Here's how the part is built. I have some questions about the finished solid (model axes, mm). Face numbers are marked on the shaded views. A direction names the side the tool comes from. Coordinates: 2 decimals unless noted, no trailing zeros. Answer in a Markdown table with one row per item. Add a question column.
Item 1: I'm going to push flat-ended pins straight in: pin 1 (1.5 mm diameter, centred on x = -9.5, z = -2.5, fed in from -Y); pin 2 (1 mm diameter, centred on y = 6.5, z = 1.5, fed in from +X); pin 3 (18 mm diameter, centred on x = 0, y = 0, fed in from -Z); pin 4 (2 mm diameter, centred on y = 20.5, z = 2, fed in from +X). Where does each tip first touch, or does it pass through?
Item 2: Imagine slicing it at A-A (x = 0). State how many separate pieces and enclosed holes the cut face has, plus the area to 3 significant figures.
Item 3: We'd pull the mould along Y, two halves only. Please class the marked faces 1 and 2: +Y half, -Y half, draft (parallel to the pull), parting line (faces both ways), or undercut.
Item 4: Which directions (+Z, -Z, +X, -X, +Y, -Y) give clear straight access to the entire face, cutting with the end or side of a thin tool? Please do the marked faces 3 and 4.
Item 5: If I drill on probe 1 along Y at (x, z) = (0, 1.25); probe 2 along Y at (x, z) = (4, 2.75); probe 3 along X at (y, z) = (16, 2), over which ranges is the centre line in solid material (lowest first)? Write a range as from..to.
from build123d import *

# Parameters (mm, degrees)
F0_R     = 11.176
F1_DEPTH = 3.5052
F2_R     = 1.778


with BuildPart() as f1:
    # F0 (on Top) → F1 (new body, symmetric)
    with BuildSketch(Plane.XY):
        with BuildLine():
            ThreePointArc((-24.84993, -0.398391), (-33.098704, -19.149794), (-12.733744, -21.369204))
            ThreePointArc((-12.733744, -21.369204), (-0.013391, -15.760536), (12.71565, -21.34946))
            ThreePointArc((12.71565, -21.34946), (33.05076, -19.116913), (24.826735, -0.385487))
            ThreePointArc((24.826735, -0.385487), (13.585768, 7.887112), (12.102172, 21.764941))
            ThreePointArc((12.102172, 21.764941), (0.004478, 38.316773), (-12.094544, 21.765913))
            ThreePointArc((-12.094544, 21.765913), (-13.5859, 7.871711), (-24.84993, -0.398391))
        make_face()
        Polygon((-26.997707, -4.0386), (-16.996384, -4.0386), (-11.995722, -12.7), (-16.996384, -21.3614), (-26.997707, -21.3614), (-31.998368, -12.7), align=None, mode=Mode.SUBTRACT)
        Polygon((16.996384, -21.3614), (11.995722, -12.7), (16.996384, -4.0386), (26.997707, -4.0386), (31.998368, -12.7), (26.997707, -21.3614), align=None, mode=Mode.SUBTRACT)
        Circle(F0_R, mode=Mode.SUBTRACT)
        Polygon((10.001323, 25.4), (5.000662, 16.7386), (-5.000662, 16.7386), (-10.001323, 25.4), (-5.000662, 34.0614), (5.000662, 34.0614), align=None, mode=Mode.SUBTRACT)
    extrude(amount=F1_DEPTH, both=True)

    # F2
    f2_edges = [f1.edges().sort_by_distance(p)[0] for p in [
        (-33.098704, -19.149794, 3.5052),
        (-0.013391, -15.760536, 3.5052),
        (-13.5859, 7.871711, 3.5052),
        (0.004478, 38.316773, 3.5052),
        (13.585768, 7.887112, 3.5052),
        (33.05076, -19.116913, 3.5052),
        (13.585768, 7.887112, -3.5052),
        (0.004478, 38.316773, -3.5052),
        (-13.5859, 7.871711, -3.5052),
        (-33.098704, -19.149794, -3.5052),
        (-0.013391, -15.760536, -3.5052),
        (33.05076, -19.116913, -3.5052),
    ]]
    fillet(f2_edges, radius=F2_R)


solid = f1.part
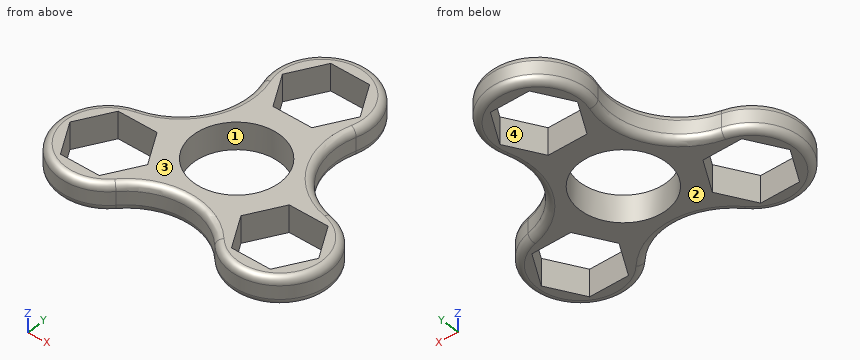
Here are the results:
| question | item | result |
|---|---|---|
| 1 | pin 1 | stops at y = -19.01 |
| 1 | pin 2 | stops at x = 14.84 |
| 1 | pin 3 | passes through |
| 1 | pin 4 | stops at x = 12.01 |
| 2 | separate pieces | 3 |
| 2 | enclosed holes | 0 |
| 2 | area | 98.3 mm2 |
| 3 | face 1 | undercut |
| 3 | face 2 | draft |
| 4 | face 3 | +Z, +X, -X, +Y, -Y |
| 4 | face 4 | +Z, -Z |
| 5 | probe 1 | y = -15.76..-11.18, 11.18..16.74, 34.06..38.32 |
| 5 | probe 2 | y = -15.9..-10.44, 10.44..16.74, 34.06..37.33 |
| 5 | probe 3 | x = -11.26..11.27 |
